The model under review builds one solid part; all positions refer to its coordinate system, in mm. Face numbers are marked on the shaded views. A direction names the side the tool comes from. Give positions to 0.01 mm unless a question says otherwise; leave off trailing zeros. Loops run counter-clockwise (first coordinate to the right, second up) from the corner with the lowest first, then second, coordinate; pieces in that order, holes last. Notation, with made-up numbers: M 17,53 L 52,53 A5 cw 52,58 Z; hole C 5.5,52.5 d5. An arc over 180 degrees is marked long. Put each result on its own line as item: value. Start each with the question number.
from build123d import *

# Parameters (mm, degrees)
SKIZZE1_R                        = 7.25
AUFSATZ_LINEAR_AUSTRAGEN1_DEPTH  = 136
SKIZZE2_R                        = 7.25
AUFSATZ_LINEAR_AUSTRAGEN2_DEPTH  = 2
SKIZZE3_R                        = 8.35
AUFSATZ_LINEAR_AUSTRAGEN3_DEPTH  = 7
AUFSATZ_LINEAR_AUSTRAGEN6_DEPTH  = 2
LINEARES_MUSTER3_COUNT           = 2
LINEARES_MUSTER3_PITCH           = 12
SKIZZE12_W                       = 32
SKIZZE12_H                       = 14
SKIZZE12_R                       = 1.6
AUFSATZ_LINEAR_AUSTRAGEN14_DEPTH = 2
SKIZZE14_R                       = 2.6
SCHNITT_LINEAR_AUSTRAGEN1_DEPTH  = 2


with BuildPart() as part:
    # Skizze1 → Aufsatz-Linear austragen1 (new body)
    with BuildSketch(Plane.XY):
        Polygon((-10.969655115, 0), (-5.484827557, -9.5), (5.484827557, -9.5), (10.969655115, 0), (5.484827557, 9.5), (-5.484827557, 9.5), align=None)
        Circle(SKIZZE1_R, mode=Mode.SUBTRACT)
    extrude(amount=AUFSATZ_LINEAR_AUSTRAGEN1_DEPTH)

    # Skizze2 → Aufsatz-Linear austragen2 (add)
    with BuildSketch(Plane.XY):
        Circle(SKIZZE2_R)
    extrude(amount=AUFSATZ_LINEAR_AUSTRAGEN2_DEPTH)

    # Skizze3 → Aufsatz-Linear austragen3 (add)
    with BuildSketch(Plane.XY.offset(133)):
        Polygon((13.279056191, 0), (6.639528096, 11.5), (-6.639528096, 11.5), (-13.279056191, 0), (-6.639528096, -11.5), (6.639528096, -11.5), align=None)
        Circle(SKIZZE3_R, mode=Mode.SUBTRACT)
    extrude(amount=AUFSATZ_LINEAR_AUSTRAGEN3_DEPTH)

    # Skizze7 → Aufsatz-Linear austragen6 (add)
    with BuildSketch(Plane.XY):
        Polygon((10.969655115, 0), (5.484827557, -9.5), (16, -9.5), align=None)
        Polygon((-5.484827557, -9.5), (-10.969655115, 0), (-16, -9.5), align=None)
    aufsatz_linear_austragen6 = extrude(amount=AUFSATZ_LINEAR_AUSTRAGEN6_DEPTH)

    # Lineares Muster3: Aufsatz-Linear austragen6 ×2
    with Locations(*[(0, 0, i * LINEARES_MUSTER3_PITCH) for i in range(1, LINEARES_MUSTER3_COUNT)]):
        add(aufsatz_linear_austragen6)

    # Skizze12 → Aufsatz-Linear austragen14 (add)
    with BuildSketch(Plane.XZ.offset(9.5)):
        with Locations((0, 7)):
            Rectangle(SKIZZE12_W, SKIZZE12_H)
        with Locations((-13, 7)):
            Circle(SKIZZE12_R, mode=Mode.SUBTRACT)
        with Locations((13, 7)):
            Circle(SKIZZE12_R, mode=Mode.SUBTRACT)
    extrude(amount=AUFSATZ_LINEAR_AUSTRAGEN14_DEPTH)

    # Skizze14 → Schnitt-Linear austragen1 (cut)
    with BuildSketch(Plane(origin=(0, 0, 0), x_dir=(-1, 0, 0), z_dir=(0, 0, -1))):
        Circle(SKIZZE14_R)
    extrude(amount=-SCHNITT_LINEAR_AUSTRAGEN1_DEPTH, mode=Mode.SUBTRACT)


solid = part.part
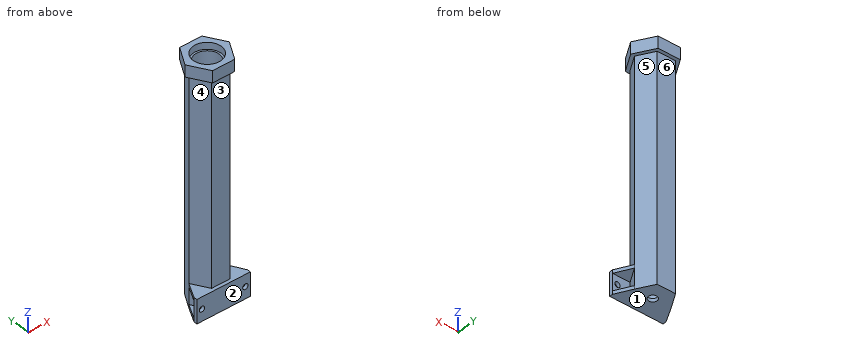
(1) Insertion check: pin 1 (12 mm diameter, centred on x = 12.5, z = 82, fed in from +Y); pin 2 (3 mm diameter, centred on y = -9, z = 79, fed in from +X); pin 3 (3 mm diameter, centred on x = -13, z = 7, fed in from -Y); pin 4 (4 mm diameter, centred on y = -9, z = 62, fed in from +X). Each pin has a flat end and moves straight along its axis. Give the tip position at first contact, or say it passes through.
(2) For the marked faces 4, 5 and 6, list the 3-axis set-ups (+Z, -Z, +X, -X, +Y, -Y) from which the entire face can be reached by the end or side of a thin tool; tool diameter is ignored.
(3) We need section B-B, the plane z = 123.5. Write out the cut boundary in (x, y).
(4) To check wall thickness, follow L1, parallel to X at y = 0, z = 137.85; L2, parallel to Y at x = 0, z = 138; L3, parallel to Z at x = -4, y = 10.25. State the ranges of each line that lie inside material, in increasing order. Write a range as [from, to].
(5) We need section A-A, the plane x = 0. Write out the cut boundary in (y, z), plus the area to 3 significant figures.
(6) Draft analysis for pull direction Z (two halves, no side actions). For the marked faces 1, 2 and 3, state which applies: +Z half, -Z half, draft (parallel to the pull), parting line (faces both ways), or undercut.
Check sheet entries:
1. pin 1: stops at y = 7.74
1. pin 2: stops at x = 6.64
1. pin 3: passes through
1. pin 4: stops at x = 6.93
2. face 4: -X, -Y
2. face 5: -Z, +X, +Y
2. face 6: -Z, +X, -X, +Y
3. outline: M -10.97,0 L -5.48,-9.5 L 5.48,-9.5 L 10.97,0 L 5.48,9.5 L -5.48,9.5 Z; hole C 0,0 d14.5
4. L1: x = [-13.28, -8.35], [8.35, 13.28]
4. L2: y = [-11.5, -8.35], [8.35, 11.5]
4. L3: z = [133, 140]
5. outline: M -11.5,0 L -2.6,0 L -2.6,2 L -7.25,2 L -7.25,136 L -8.35,136 L -8.35,140 L -11.5,140 L -11.5,133 L -9.5,133 L -9.5,14 L -11.5,14 Z; M 2.6,0 L 9.5,0 L 9.5,133 L 11.5,133 L 11.5,140 L 8.35,140 L 8.35,136 L 7.25,136 L 7.25,2 L 2.6,2 Z
5. area: 696 mm²
6. face 1: -Z half
6. face 2: draft
6. face 3: undercut
